from build123d import *

# Parameters (mm, degrees)
F0_W     = 10.000005
F0_H     = 101.6
F1_DEPTH = 3.999992
F2_W     = 3.545
F2_H     = 83.283524
F3_DEPTH = 8.000009
F4_W     = 10.000005
F4_H     = 5.709733
F4_H_2   = 5.71377
F5_DEPTH = 1.6764
F6_DEPTH = 1.6764
F7_R     = 1.7526
F8_DEPTH = 25.4
F9_R     = 5.08
F10_R    = 5.08
F11_R    = 1.27
F12_R    = 5.08
F13_R    = 5.08
F14_R    = 1.27


with BuildPart() as f1:
    # F0 (on Top) → F1 (new body)
    with BuildSketch(Plane.XY):
        with Locations((-0.961494, 14.724417)):
            Rectangle(F0_W, F0_H)
    extrude(amount=F1_DEPTH)

    # F2 (on face) → F3 (join)
    with BuildSketch(Plane.XY.offset(3.999992)):
        with Locations((2.266009, 14.282725)):
            Rectangle(F2_W, F2_H)
        with Locations((-4.188996, 14.282725)):
            Rectangle(F2_W, F2_H)
    extrude(amount=F3_DEPTH)

    # F4 (on face) → F5 (cut)
    with BuildSketch(Plane.XY.offset(3.999992)):
        with Locations((-0.961494, 58.779353)):
            Rectangle(F4_W, F4_H)
        with Locations((-0.961494, -30.215922)):
            Rectangle(F4_W, F4_H_2)
    extrude(amount=-F5_DEPTH, mode=Mode.SUBTRACT)

    # F4 (on face) → F6 (cut)
    with BuildSketch(Plane.XY.offset(3.999992)):
        with Locations((-0.961494, 58.779353)):
            Rectangle(F4_W, F4_H)
        with Locations((-0.961494, -30.215922)):
            Rectangle(F4_W, F4_H_2)
    extrude(amount=-F6_DEPTH, mode=Mode.SUBTRACT)

    # F7 (on face) → F8 (cut)
    with BuildSketch(Plane.YZ.offset(4.038509)):
        with Locations((-12.17894, 8.000104)):
            Circle(F7_R)
        with Locations((43.18684, 8.000104)):
            Circle(F7_R)
    extrude(amount=-F8_DEPTH, mode=Mode.SUBTRACT)

    # F9
    f9_edges = [f1.edges().sort_by_distance(p)[0] for p in [
        (-4.188996, -27.359037, 12.000001),
    ]]
    fillet(f9_edges, radius=F9_R)

    # F10
    f10_edges = [f1.edges().sort_by_distance(p)[0] for p in [
        (2.266009, -27.359037, 12.000001),
    ]]
    fillet(f10_edges, radius=F10_R)

    # F11
    f11_edges = [f1.edges().sort_by_distance(p)[0] for p in [
        (-0.961494, -36.075583, 3.999992),
    ]]
    fillet(f11_edges, radius=F11_R)

    # F12
    f12_edges = [f1.edges().sort_by_distance(p)[0] for p in [
        (2.266009, 55.924487, 12.000001),
    ]]
    fillet(f12_edges, radius=F12_R)

    # F13
    f13_edges = [f1.edges().sort_by_distance(p)[0] for p in [
        (-4.188996, 55.924487, 12.000001),
    ]]
    fillet(f13_edges, radius=F13_R)

    # F14
    f14_edges = [f1.edges().sort_by_distance(p)[0] for p in [
        (-0.961494, 65.524417, 3.999992),
    ]]
    fillet(f14_edges, radius=F14_R)


solid = f1.part
Model file for the job. Use its own axes, mm. A direction names the side the tool comes from. Round coordinates to 2 decimals unless told otherwise and drop trailing zeros. Order: outer loops, then holes, each group sorted by start corner. A loop starts at its lowest first (then second) coordinate and runs counter-clockwise, first axis right, second up.
(1) Band-saw the part on B-B (y = -11.5). List the corners of the cut face in (x, z).
(2) Drill centre lines: line 1 (Z direction, x = -4, y = 43); line 2 (X direction, y = -16.5, z = 8); line 3 (Y direction, x = 2.75, z = 9.5). Where is each one in solid material? Low to high.
(3) Pull direction Z, two halves, no side cores. Call faces 1 (the face through (2.29, -25.91, 10.47)), 2 (the face through (-1, 65.524, 1)), 3 (the face through (-4.2, -10.5, 8.5)): released by +Z, released by -Z, zero draft, split by the parting line, or undercut.
(4) 3-axis set-ups, long thin cutter, end or side, ignore diameter. For faces 4 (the face through (2.291, 41.436, 8.077)), 5 (the face through (-4, 55.924, 5)), 6 (the face through (-5.961, 14, 8)), 7 (the face through (-1, 15, 4)), 8 (the face through (-1, -33.073, 3)): which of +Z, -Z, +X, -X, +Y, -Y reach the whole face in a straight line?
(5) Band-saw the part on C-C (y = 52). List the corners of the cut face in (x, z), then the cut area to 3 significant figures.
(6) Band-saw the part on A-A (x = -1). List the corners of the cut face in (y, z).
(7) Pin check, flat tips, straight feed: pin 1 (0.9 mm diameter, centred on x = 1.5, y = -34.5, fed in from +Z); pin 2 (3 mm diameter, centred on x = 2, z = 6, fed in from +Y); pin 3 (1.7 mm diameter, centred on x = 1.5, y = 60, fed in from +Z). Stop position of each tip, or through.
Verdict:
1. outline: (-5.96, 0) - (4.04, 0) - (4.04, 6.38) - (0.49, 6.38) - (0.49, 4) - (-2.42, 4) - (-2.42, 6.38) - (-5.96, 6.38) - close; (-5.96, 9.62) - (-2.42, 9.62) - (-2.42, 12) - (-5.96, 12) - close; (0.49, 9.62) - (4.04, 9.62) - (4.04, 12) - (0.49, 12) - close
2. line 1: z = 0 to 6.26, 9.74 to 12
2. line 2: x = -5.96 to -2.42, 0.49 to 4.04
2. line 3: y = -26.66 to -13.09, -11.27 to 42.28, 44.09 to 55.22
3. face 1: released by +Z
3. face 2: zero draft
3. face 3: undercut
4. face 4: +X, -X
4. face 5: +Z, +X, -X, +Y
4. face 6: +Z, -Z, -X, +Y, -Y
4. face 7: +Z, +Y, -Y
4. face 8: +Z, +X, -X
5. outline: (-5.96, 0) - (4.04, 0) - (4.04, 11.87) - (0.49, 11.87) - (0.49, 4) - (-2.42, 4) - (-2.42, 11.87) - (-5.96, 11.87) - close
5. area: 95.8 mm2
6. outline: (-36.08, 0) - (65.52, 0) - (65.52, 2.73) arc R1.27 ccw to (64.25, 4) - (61.63, 4) - (61.63, 2.32) - (55.92, 2.32) - (55.92, 4) - (-27.36, 4) - (-27.36, 2.32) - (-33.07, 2.32) - (-33.07, 4) - (-34.81, 4) arc R1.27 ccw to (-36.08, 2.73) - close
7. pin 1: stops at z = 4
7. pin 2: stops at y = 55.92
7. pin 3: stops at z = 2.32
